Verification items for the finished model (mm, model axes). A direction names the side the tool comes from. Coordinates: 2 decimals unless noted, no trailing zeros. Order: outer loops, then holes, each group sorted by start corner. A loop starts at its lowest first (then second) coordinate and runs counter-clockwise, first axis right, second up.
Q1. Set-up check for faces 3 (the cylindrical face through (-4, 0, 10)), 4 (the flat face through (0, 7.1, 4)), 5 (the cylindrical face through (4.09, -0.04, 2.16)), 6 (the flat face through (8, 1.148, 10)): record each of +Z, -Z, +X, -X, +Y, -Y from which the full face is reachable in a straight line by a thin tool's end or side.
Q2. Cross-section at D-D, the plane x = 4.5. Record the boundary of the cut face in (y, z).
Q3. Cross-section at C-C, the plane z = 10.5. Record the boundary of the cut face in (x, y), and give its area (3 significant figures).
Q4. Draft check along Z on faces 1 (the flat face through (2.646, 4.5, 7.5)), 2 (the flat face through (0, 7, 10)). Enter one of: pulls with the +Z half, pulls with the -Z half, needs draft (parallel to the pull), parting line crosses it, or undercut.
Q5. Depth check by flat-ended pin: P1, Ø5, axis at y = 1.5, z = 3, coming from the -X side; P2, Ø6, axis at y = 2.5, z = 2, coming from the +X side; P3, Ø2.5, axis at x = 8.5, z = 11.5, coming from the -Y side; P4, Ø2.5, axis at x = 9, z = 10.5, coming from the +Y side. Enter the tip coordinate at first touch or a pass-through.
Q6. Thickness scan on line 1 (Y direction, x = 7.25, z = 8.25); line 2 (Z direction, x = 0.75, y = -6.75); line 3 (Y direction, x = 2, z = 4.75). Record the ranges inside material, lowest first.
Q7. Cross-section at B-B, the plane y = 4. Record the boundary of the cut face in (x, z), and give its area (3 significant figures).
Q8. Cross-section at A-A, the plane x = 7.75. Record the boundary of the cut face in (y, z).
from build123d import *

# Parameters (mm, degrees)
SKETCH_1_W               = 16
SKETCH_1_H               = 20
EXTRUDE_1_DEPTH          = 7
CUT_EXTRUDE_1_DEPTH      = 15
CUT_EXTRUDE_3_DEPTH      = 15.594519519
SKETCH_6_W               = 5.291502622
SKETCH_6_H               = 4
EXTRUDE_2_DEPTH          = 1
CUT_EXTRUDE_5_DEPTH      = 17.338184405
CUT_EXTRUDE_5_DEPTH_BACK = 17.338184405
SKETCH_7_W               = 2.2
SKETCH_7_H               = 14.2
SKETCH_8_R               = 4.915012662
EXTRUDE_3_DEPTH          = 1.5
SKETCH_9_R               = 7
SKETCH_9_R_2             = 4
EXTRUDE_4_DEPTH          = 5
SKETCH_10_W              = 5.291502622
SKETCH_10_H              = 4
SKETCH_10_W_2            = 5.341465502
SKETCH_10_H_2            = 1.894443453
EXTRUDE_5_DEPTH          = 5
FILLET_1_R               = 1
EXTRUDE_6_DEPTH          = 5
CUT_EXTRUDE_6_DEPTH      = 21.622580814
CUT_EXTRUDE_6_DEPTH_BACK = 5
SKETCH_12_W              = 10.898323227
SKETCH_12_H              = 2
SKETCH_13_R              = 1.6
CUT_EXTRUDE_7_DEPTH      = 23.232652551


with BuildPart() as part:
    # 草图1 → 凸台-拉伸1 (new body)
    with BuildSketch(Plane.XY):
        Rectangle(SKETCH_1_W, SKETCH_1_H)
    extrude(amount=EXTRUDE_1_DEPTH)

    # 草图2 → 切除-拉伸1 (cut)
    with BuildSketch(Plane.XY.offset(7)):
        with BuildLine():
            Line((-2.645751311, 3), (2.645751311, 3))
            ThreePointArc((2.645751311, 3), (4.091798312, -0.088548302), (2.695714191, -3.2))
            Line((2.695714191, -3.2), (-2.695714191, -3.2))
            ThreePointArc((-2.695714191, -3.2), (-4.091798312, -0.088548302), (-2.645751311, 3))
        make_face()
    extrude(amount=-CUT_EXTRUDE_1_DEPTH, mode=Mode.SUBTRACT)

    # 草图4 → 切除-拉伸3 (cut, through all)
    with BuildSketch(Plane.XY.offset(7)):
        with BuildLine():
            Line((-3.842719282, 10), (-8, 10))
            Line((-8, 10), (-8, -10))
            Line((-8, -10), (-3.842719282, -10))
            ThreePointArc((-3.842719282, -10), (-7.5, 0), (-3.842719282, 10))
        make_face()
        with BuildLine():
            Line((3.842719282, 10), (8, 10))
            Line((8, 10), (8, -10))
            Line((8, -10), (3.842719282, -10))
            ThreePointArc((3.842719282, -10), (7.5, 0), (3.842719282, 10))
        make_face()
    extrude(amount=-CUT_EXTRUDE_3_DEPTH, mode=Mode.SUBTRACT)

    # 草图6 → 凸台-拉伸2 (add)
    with BuildSketch(Plane.XY.offset(7)):
        with Locations((0, 5)):
            Rectangle(SKETCH_6_W, SKETCH_6_H)
    extrude(amount=EXTRUDE_2_DEPTH)

    # 草图7 → 切除-拉伸5 (cut, two sides: drawn at the far end of the back side and taken through both)
    with BuildSketch(Plane.ZY.offset(2.645751311).offset(-CUT_EXTRUDE_5_DEPTH_BACK)):
        with Locations((3.9, 0)):
            Rectangle(SKETCH_7_W, SKETCH_7_H)
    extrude(amount=CUT_EXTRUDE_5_DEPTH + CUT_EXTRUDE_5_DEPTH_BACK, mode=Mode.SUBTRACT)

    # 草图8 → 凸台-拉伸3 (add)
    with BuildSketch(Plane(origin=(0, 0, 0), x_dir=(-1, 0, 0), z_dir=(0, 0, -1))):
        Circle(SKETCH_8_R)
    extrude(amount=-EXTRUDE_3_DEPTH)

    # 草图9 → 凸台-拉伸4 (add)
    with BuildSketch(Plane.XY.offset(8)):
        with Locations(Location((0, 0, 0), (0, 0, 112.207654299))):
            Circle(SKETCH_9_R)
        with Locations(Location((0, 0, 0), (0, 0, 131.409622109))):
            Circle(SKETCH_9_R_2, mode=Mode.SUBTRACT)
    extrude(amount=EXTRUDE_4_DEPTH)

    # 草图10 → 凸台-拉伸5 (add)
    with BuildSketch(Plane.XY.offset(8)):
        with Locations((0, 5)):
            Rectangle(SKETCH_10_W, SKETCH_10_H)
        with Locations((0.02498144, -4.147221726)):
            Rectangle(SKETCH_10_W_2, SKETCH_10_H_2)
    extrude(amount=EXTRUDE_5_DEPTH)

    # 圆角1
    # the kernel refuses this fillet: 1 mm, written as the material it takes off along each edge
    with BuildSketch(Plane(origin=(2.645751311, 7, 7), x_dir=(-1, 0, 0), z_dir=(0, 0, 1))) as fillet_1_piece_1_section:
        with BuildLine():
            CenterArc((FILLET_1_R, FILLET_1_R), FILLET_1_R, 180, 90)
            Line((0, FILLET_1_R), (0, 0))
            Line((0, 0), (FILLET_1_R, 0))
        make_face()
    fillet_1_piece_1 = extrude(amount=8.5, mode=Mode.PRIVATE)
    fillet_1_piece_1 = split(fillet_1_piece_1, bisect_by=Plane(origin=(2.390465062, 6.836939251, 8), z_dir=(0, 0, -1)), keep=Keep.TOP, mode=Mode.PRIVATE)
    fillet_1_piece_1 = fillet_1_piece_1 - Plane(origin=(0, 0, 7.5), x_dir=(-0.3779644730157475, 0.9258200997698897, 0), z_dir=(0, 0, -1)) * Cylinder(7, 21, mode=Mode.PRIVATE)
    add(fillet_1_piece_1, mode=Mode.SUBTRACT)
    with BuildSketch(Plane(origin=(2.645751311, 7, 7), x_dir=(-1, 0, 0), z_dir=(0, 0, 1))) as fillet_1_piece_2_section:
        with BuildLine():
            CenterArc((FILLET_1_R, FILLET_1_R), FILLET_1_R, 180, 90)
            Line((0, FILLET_1_R), (0, 0))
            Line((0, 0), (FILLET_1_R, 0))
        make_face()
    fillet_1_piece_2 = extrude(amount=8.5, mode=Mode.PRIVATE)
    fillet_1_piece_2 = split(fillet_1_piece_2, bisect_by=Plane(origin=(2.615865348, 6.342822841, 8), z_dir=(0, 0, -1)), keep=Keep.TOP, mode=Mode.PRIVATE)
    fillet_1_piece_2 = fillet_1_piece_2 & Plane(origin=(0, 0, 7.5), x_dir=(-0.3779644730157475, 0.9258200997698897, 0), z_dir=(0, 0, -1)) * Cylinder(7, 21, mode=Mode.PRIVATE)
    add(fillet_1_piece_2, mode=Mode.SUBTRACT)
    with BuildSketch(Plane(origin=(2.645751311, 7, 7), x_dir=(-1, 0, 0), z_dir=(0, 0, 1))) as fillet_1_piece_3_section:
        with BuildLine():
            CenterArc((FILLET_1_R, FILLET_1_R), FILLET_1_R, 180, 90)
            Line((0, FILLET_1_R), (0, 0))
            Line((0, 0), (FILLET_1_R, 0))
        make_face()
    fillet_1_piece_3 = extrude(amount=8.5, mode=Mode.PRIVATE)
    fillet_1_piece_3 = split(fillet_1_piece_3, bisect_by=Plane(origin=(2.390465062, 6.836939251, 8), z_dir=(0, 0, 1)), keep=Keep.TOP, mode=Mode.PRIVATE)
    fillet_1_piece_3 = fillet_1_piece_3 - Plane(origin=(0, 0, 11.75), x_dir=(-0.3779644730157475, 0.9258200997698897, 0), z_dir=(0, 0, -1)) * Cylinder(7, 21, mode=Mode.PRIVATE)
    add(fillet_1_piece_3, mode=Mode.SUBTRACT)
    with BuildSketch(Plane(origin=(-2.645751311, 7, 7), x_dir=(0, -1, 0), z_dir=(0, 0, 1))) as fillet_1_piece_4_section:
        with BuildLine():
            CenterArc((FILLET_1_R, FILLET_1_R), FILLET_1_R, 180, 90)
            Line((0, FILLET_1_R), (0, 0))
            Line((0, 0), (FILLET_1_R, 0))
        make_face()
    fillet_1_piece_4 = extrude(amount=8.5, mode=Mode.PRIVATE)
    fillet_1_piece_4 = fillet_1_piece_4 & Plane(origin=(0, 0, 7.5), x_dir=(-0.3779644730157475, 0.9258200997698897, 0), z_dir=(0, 0, -1)) * Cylinder(7, 21, mode=Mode.PRIVATE)
    fillet_1_piece_4 = split(fillet_1_piece_4, bisect_by=Plane(origin=(-2.615865348, 6.342822841, 8), z_dir=(0, 0, -1)), keep=Keep.TOP, mode=Mode.PRIVATE)
    add(fillet_1_piece_4, mode=Mode.SUBTRACT)
    with BuildSketch(Plane(origin=(-2.645751311, 7, 7), x_dir=(0, -1, 0), z_dir=(0, 0, 1))) as fillet_1_piece_5_section:
        with BuildLine():
            CenterArc((FILLET_1_R, FILLET_1_R), FILLET_1_R, 180, 90)
            Line((0, FILLET_1_R), (0, 0))
            Line((0, 0), (FILLET_1_R, 0))
        make_face()
    fillet_1_piece_5 = extrude(amount=8.5, mode=Mode.PRIVATE)
    fillet_1_piece_5 = fillet_1_piece_5 - Plane(origin=(0, 0, 7.5), x_dir=(-0.3779644730157475, 0.9258200997698897, 0), z_dir=(0, 0, -1)) * Cylinder(7, 21, mode=Mode.PRIVATE)
    fillet_1_piece_5 = split(fillet_1_piece_5, bisect_by=Plane(origin=(-2.390465062, 6.836939251, 8), z_dir=(0, 0, -1)), keep=Keep.TOP, mode=Mode.PRIVATE)
    add(fillet_1_piece_5, mode=Mode.SUBTRACT)
    with BuildSketch(Plane(origin=(-2.645751311, 7, 7), x_dir=(0, -1, 0), z_dir=(0, 0, 1))) as fillet_1_piece_6_section:
        with BuildLine():
            CenterArc((FILLET_1_R, FILLET_1_R), FILLET_1_R, 180, 90)
            Line((0, FILLET_1_R), (0, 0))
            Line((0, 0), (FILLET_1_R, 0))
        make_face()
    fillet_1_piece_6 = extrude(amount=8.5, mode=Mode.PRIVATE)
    fillet_1_piece_6 = fillet_1_piece_6 - Plane(origin=(0, 0, 11.75), x_dir=(-0.3779644730157475, 0.9258200997698897, 0), z_dir=(0, 0, -1)) * Cylinder(7, 21, mode=Mode.PRIVATE)
    fillet_1_piece_6 = split(fillet_1_piece_6, bisect_by=Plane(origin=(-2.390465062, 6.836939251, 8), z_dir=(0, 0, 1)), keep=Keep.TOP, mode=Mode.PRIVATE)
    add(fillet_1_piece_6, mode=Mode.SUBTRACT)

    # 草图11 → 凸台-拉伸6 (add)
    with BuildSketch(Plane.XY.offset(13)):
        Polygon((12.501633471, 1), (12.501633471, -1), (12.501633471, -3), (5.400773292, -3), (5.400773292, -1), (5.400773292, 1), (5.400773292, 3), (12.501633471, 3), align=None)
    extrude(amount=-EXTRUDE_6_DEPTH)

    # 草图12 → 切除-拉伸6 (cut, two sides: drawn at the far end of the back side and taken through both)
    with BuildSketch(Plane.XY.offset(13).offset(-CUT_EXTRUDE_6_DEPTH_BACK)):
        with Locations((7.052471858, 0.148280364)):
            Rectangle(SKETCH_12_W, SKETCH_12_H)
    extrude(amount=CUT_EXTRUDE_6_DEPTH + CUT_EXTRUDE_6_DEPTH_BACK, mode=Mode.SUBTRACT)

    # 草图13 → 切除-拉伸7 (cut, through all)
    with BuildSketch(Plane(origin=(0, 3, 0), x_dir=(1, 0, 0), z_dir=(0, 1, 0))):
        with Locations(Location((9.82455532, -10.5, 0), (0, 0, 270))):
            Circle(SKETCH_13_R)
    extrude(amount=-CUT_EXTRUDE_7_DEPTH, mode=Mode.SUBTRACT)


solid = part.part
Check values:
1. face 3: +Z
1. face 4: +X, -X
1. face 5: none
1. face 6: +Z, +X
2. outline: (-9.17, 0) - (9.17, 0) - (9.17, 7) - (-9.17, 7) - close; (-5.36, 8) - (-0.85, 8) - (-0.85, 13) - (-5.36, 13) - close; (1.15, 8) - (5.36, 8) - (5.36, 13) - (1.15, 13) - close; hole (-7.1, 2.8) - (7.1, 2.8) - (7.1, 5) - (-7.1, 5) - close
3. outline: (-2.65, 3) - (2.65, 3) arc R4 cw to (3.83, 1.15) - (8.22, 1.15) - (8.22, 3) - (6.32, 3) arc R7 ccw to (2.48, 6.54) arc R1 ccw to (1.65, 7) - (-1.65, 7) arc R1 ccw to (-2.48, 6.54) arc R7 ccw (long way) to (6.32, -3) - (8.22, -3) - (8.22, -0.85) - (3.91, -0.85) arc R4 cw to (2.4, -3.2) - (-2.4, -3.2) arc R4 cw to start; (11.42, -3) - (12.5, -3) - (12.5, -0.85) - (11.42, -0.85) - close; (11.42, 1.15) - (12.5, 1.15) - (12.5, 3) - (11.42, 3) - close
3. area: 115 mm2
4. face 1: undercut
4. face 2: needs draft
5. P1: stops at x = -7.5
5. P2: stops at x = 7.5
5. P3: stops at y = -3
5. P4: stops at y = 3
6. line 1: y = -3 to -0.85, 1.15 to 3
6. line 2: z = 0 to 2.8, 5 to 7, 8 to 13
6. line 3: y = -10 to -7.1, 7.1 to 10
7. outline: (-6.97, 0) - (6.97, 0) - (6.97, 2.8) - (-6.97, 2.8) - close; (-6.97, 5) - (6.97, 5) - (6.97, 7) - (2.65, 7) - (2.65, 8) - (5.74, 8) - (5.74, 13) - (-5.74, 13) - (-5.74, 8) - (-2.65, 8) - (-2.65, 7) - (-6.97, 7) - close
7. area: 130 mm2
8. outline: (-3, 8) - (-0.85, 8) - (-0.85, 13) - (-3, 13) - close; (1.15, 8) - (3, 8) - (3, 13) - (1.15, 13) - close
